Part model, mm, in its own coordinate system. A direction names the side the tool comes from. Coordinates: 2 decimals unless noted, no trailing zeros. Write each loop counter-clockwise with the first axis right and the second up, starting at its lowest first coordinate (ties: lowest second). Pieces come first, ordered by that corner, then holes. Notation, with made-up numbers: (32.25, -31.75) - (59.25, -31.75) arc R21 ccw to (59.25, -14.75) - close; hole circle Ø5 at (-23.75, 66.25). An arc over 180 degrees is marked (long way). Write each question's results on one line, items separated by ' | '.
from build123d import *

# Parameters (mm, degrees)
F0_R           = 330.2
F0_R_2         = 266.7
F1_DEPTH       = 25.4
F1_DEPTH_BACK  = 25.4
F3_R           = 44.45
F3_R_2         = 38.1
F4_DEPTH       = 6.35
F3_R_3         = 31.75
F5_DEPTH       = 12.7
F3_R_4         = 25.4
F6_DEPTH       = 19.05
F3_R_5         = 19.05
F7_DEPTH       = 25.4
F9_R           = 63.5
F10_DEPTH      = 6.35
F3_R_6         = 6.35
F11_DEPTH      = 25.4
F11_DEPTH_BACK = 76.2
F12_R          = 19.05
F12_R_2        = 2.54
F13_DEPTH      = 25.4
F14_DEPTH      = 107.951
F16_DEPTH      = 12.7
F16_DEPTH_BACK = 12.7
F17_DEPTH      = 107.951
F18_R          = 25.4
F19_DEPTH      = 25.4
F19_DEPTH_BACK = 25.4
F20_R          = 304.0753924765
F20_R_2        = 266.7
F21_DEPTH      = 12.7
F22_R          = 304.0753924765
F22_R_2        = 266.7
F23_DEPTH      = 12.7


with BuildPart() as f1:
    # F0 (on Front) → F1 (new body, two sides)
    with BuildSketch(Plane.XZ) as f1_sk:
        Circle(F0_R)
        Circle(F0_R_2, mode=Mode.SUBTRACT)
    extrude(amount=F1_DEPTH)
    extrude(f1_sk.sketch, amount=-F1_DEPTH_BACK)



with BuildPart() as f4:
    # F3 (on offset) → F4 (new body)
    with BuildSketch(Plane.XZ.offset(38.1)):
        Circle(F3_R)
        Circle(F3_R_2, mode=Mode.SUBTRACT)
    extrude(amount=F4_DEPTH)

    # F3 (on offset) → F5 (join)
    with BuildSketch(Plane.XZ.offset(38.1)):
        Circle(F3_R_2)
        Circle(F3_R_3, mode=Mode.SUBTRACT)
    extrude(amount=F5_DEPTH)

    # F3 (on offset) → F6 (join)
    with BuildSketch(Plane.XZ.offset(38.1)):
        Circle(F3_R_3)
        Circle(F3_R_4, mode=Mode.SUBTRACT)
    extrude(amount=F6_DEPTH)

    # F3 (on offset) → F7 (join)
    with BuildSketch(Plane.XZ.offset(38.1)):
        Circle(F3_R_4)
        Circle(F3_R_5, mode=Mode.SUBTRACT)
    extrude(amount=F7_DEPTH)



with BuildPart() as f10:
    # F9 (on offset) → F10 (new body)
    with BuildSketch(Plane(origin=(0, 38.1, 0), x_dir=(-1, 0, 0), z_dir=(0, 1, 0))):
        Circle(F9_R)
    extrude(amount=F10_DEPTH)

    # F3 (on offset) → F11 (join, two sides)
    with BuildSketch(Plane.XZ.offset(38.1)) as f11_sk:
        Circle(F3_R_6)
    extrude(amount=F11_DEPTH)
    extrude(f11_sk.sketch, amount=-F11_DEPTH_BACK)


with BuildPart() as f4_1:
    add(f4.part)

    add(f10.part)  # F13 merges F10
    # F12 (on face) → F13 (join)
    with BuildSketch(Plane.XZ.offset(63.5)):
        Circle(F12_R)
        Circle(F12_R_2, mode=Mode.SUBTRACT)
    extrude(amount=-F13_DEPTH)

    # F12 (on face) → F14 (cut, through all)
    with BuildSketch(Plane.XZ.offset(63.5)):
        Circle(F12_R_2)
    extrude(amount=-F14_DEPTH, mode=Mode.SUBTRACT)


with BuildPart() as f1_1:
    add(f1.part)

    add(f4_1.part)  # F16 merges F4
    # F15 (on Front) → F16 (join, two sides)
    with BuildSketch(Plane.XZ) as f16_sk:
        with BuildLine():
            Line((304.8, 2.54), (5.8198711326, 2.54))
            ThreePointArc((5.8198711326, 2.54), (6.2160550871, 1.2973662374), (6.35, 0))
            ThreePointArc((6.35, 0), (6.2160550871, -1.2973662374), (5.8198711326, -2.54))
            Line((5.8198711326, -2.54), (304.8, -2.54))
            Line((304.8, -2.54), (304.8, 2.54))
        make_face()
        with BuildLine():
            ThreePointArc((-5.8198711326, -2.54), (-6.35, 0), (-5.8198711326, 2.54))
            Line((-5.8198711326, 2.54), (-304.8, 2.54))
            Line((-304.8, 2.54), (-304.8, -2.54))
            Line((-304.8, -2.54), (-5.8198711326, -2.54))
        make_face()
    extrude(amount=F16_DEPTH)
    extrude(f16_sk.sketch, amount=-F16_DEPTH_BACK)

    # F12 (on face) → F17 (cut, through all)
    with BuildSketch(Plane.XZ.offset(63.5)):
        Circle(F12_R_2)
    extrude(amount=-F17_DEPTH, mode=Mode.SUBTRACT)

    # F18 (on Front) → F19 (join, two sides)
    with BuildSketch(Plane.XZ) as f19_sk:
        Circle(F18_R)
    extrude(amount=F19_DEPTH)
    extrude(f19_sk.sketch, amount=-F19_DEPTH_BACK)

    # F20 (on face) → F21 (cut)
    with BuildSketch(Plane.XZ.offset(25.4)):
        Circle(F20_R)
        Circle(F20_R_2, mode=Mode.SUBTRACT)
    extrude(amount=-F21_DEPTH, mode=Mode.SUBTRACT)

    # F22 (on face) → F23 (cut)
    with BuildSketch(Plane(origin=(0, 25.4, 0), x_dir=(-1, 0, 0), z_dir=(0, 1, 0))):
        Circle(F22_R)
        Circle(F22_R_2, mode=Mode.SUBTRACT)
    extrude(amount=-F23_DEPTH, mode=Mode.SUBTRACT)


solid = f1_1.part
(1) Saw through at C-C on x = 251.5. Write the cut outline in (y, z).
Return value:
outline: (-25.4, -213.96) - (25.4, -213.96) - (25.4, -170.91) - (12.7, -170.91) - (12.7, -88.75) - (-12.7, -88.75) - (-12.7, -170.91) - (-25.4, -170.91) - close; (-25.4, 170.91) - (-12.7, 170.91) - (-12.7, 88.75) - (12.7, 88.75) - (12.7, 170.91) - (25.4, 170.91) - (25.4, 213.96) - (-25.4, 213.96) - close; (-12.7, -2.54) - (12.7, -2.54) - (12.7, 2.54) - (-12.7, 2.54) - close
(2) Two-plate mould, pull along X, no slides. Class faces 5 (the flat face through (33, -44.45, 20)), 6 (the cylindrical face through (42.397, -41.231, 13.352)), 7 (the cylindrical face through (-5.829, 0.178, -266.636)), 8 (the flat face through (148, 0, 2.54)): released by +X, released by -X, zero draft, split by the parting line, or undercut.
Return value:
face 5: zero draft | face 6: split by the parting line | face 7: undercut | face 8: undercut
(3) 3-axis set-ups, long thin cutter, end or side, ignore diameter. For faces 1 (the flat face through (5, 25.4, -5)), 2 (the cylindrical face through (5.829, 0.178, 266.636)), 3 (the cylindrical face through (-5.506, -60.281, -24.796)), 4 (the cylindrical face through (-163.469, 19.139, 256.398)): which of +Z, -Z, +X, -X, +Y, -Y reach the whole face in a straight line?
Return value:
face 1: none | face 2: +Y, -Y | face 3: -Y | face 4: +Y
(4) Saw through at B-B on z = -149.5. Write the cut outline in (x, y).
Return value:
outline: (-294.42, -25.4) - (-264.79, -25.4) - (-264.79, -12.7) - (-220.86, -12.7) - (-220.86, 12.7) - (-264.79, 12.7) - (-264.79, 25.4) - (-294.42, 25.4) - close; (220.86, -12.7) - (264.79, -12.7) - (264.79, -25.4) - (294.42, -25.4) - (294.42, 25.4) - (264.79, 25.4) - (264.79, 12.7) - (220.86, 12.7) - close
(5) Saw through at A-A on x = -252. Write the cut outline in (y, z).
Return value:
outline: (-25.4, -213.37) - (25.4, -213.37) - (25.4, -170.17) - (12.7, -170.17) - (12.7, -87.32) - (-12.7, -87.32) - (-12.7, -170.17) - (-25.4, -170.17) - close; (-25.4, 170.17) - (-12.7, 170.17) - (-12.7, 87.32) - (12.7, 87.32) - (12.7, 170.17) - (25.4, 170.17) - (25.4, 213.37) - (-25.4, 213.37) - close; (-12.7, -2.54) - (12.7, -2.54) - (12.7, 2.54) - (-12.7, 2.54) - close
(6) Flat gauge pins, fed straight in: P1, Ø2.5, axis at x = -134.5, z = 1, coming from the +Y side; P2, Ø7.5, axis at x = 131, y = 3.5, coming from the -Z side; P3, Ø12.5, axis at x = -143, y = -2, coming from the +Z side; P4, Ø6.5, axis at x = 0, z = 0, coming from the -Y side. Where does each tip first touch, or does it go through?
Return value:
P1: stops at y = 12.7 | P2: stops at z = -304.7 | P3: stops at z = 300.55 | P4: stops at y = -63.5
(7) Wall check: line 1 (Z direction, x = 0, y = 20); line 2 (Z direction, x = 0, y = -50); line 3 (Z direction, x = 120, y = -4.5). Give the ranges that are in metal, low to high. Write a range as from..to.
Return value:
line 1: z = -330.2..-304.08, -25.4..25.4, 304.08..330.2 | line 2: z = -38.1..-2.54, 2.54..38.1 | line 3: z = -307.62..-238.18, -2.54..2.54, 238.18..307.62
